Verification items for the finished model (mm, model axes). Coordinates: 2 decimals unless noted, no trailing zeros. Order: outer loops, then holes, each group sorted by start corner. A loop starts at its lowest first (then second) coordinate and runs counter-clockwise, first axis right, second up. Notation, with made-up numbers: M -24.5,-14.5 L 14.5,-14.5 A15 cw 14.5,10.5 Z; hole C -18.5,-26.5 d6. An arc over 180 degrees is marked long. Return JSON: item names as keys, results as strings. Group by question number.
1. Material ranges on line 1 along Y through (x, z) = (2, 17); line 2 along Y through (x, z) = (-54.5, 13.25); line 3 along Y through (x, z) = (-155.5, 5.5), recorded low to high.
2. Section check D-D, the plane x = 74. Record the cut outline in (y, z), plus the area to 3 significant figures.
3. Section check C-C, the plane x = 7. Record the cut outline in (y, z).
4. Section check A-A, the plane z = 10.5. Record the cut outline in (x, y).
5. Gauge pin test, flat end, axial feed: pin 1 (4 mm diameter, centred on x = -7, z = 16.5, fed in from -Y). Record the tip position at first contact, or that the pin passes through.
6. Section check B-B, the plane y = 96.5. Record the cut outline in (x, z), plus the area to 3 significant figures.
```python
from build123d import *

# Parameters (mm, degrees)
F0_W     = 400
F0_H     = 350
F1_DEPTH = 19
F2_W     = 400
F2_H     = 350
F3_DEPTH = 19.001
F5_DEPTH = 19.001


with BuildPart() as f1:
    # F0 (on Top) → F1 (new body)
    with BuildSketch(Plane.XY):
        with Locations((0, -4.671676)):
            Rectangle(F0_W, F0_H)
    extrude(amount=F1_DEPTH)

    # F2 (on face) → F3 (cut, through all)
    with BuildSketch(Plane.XY.offset(19)):
        with Locations((0, -4.671676)):
            Rectangle(F2_W, F2_H)
        with BuildLine():
            ThreePointArc((192.000002, -145.333663), (0.340362, -123.303121), (-191.445097, -144.210055))
            Line((-191.445097, -144.210055), (-191.445097, 137.21716))
            ThreePointArc((-191.445097, 137.21716), (0.366935, 114.931669), (192.000002, 138.707012))
            Line((192.000002, 138.707012), (192.000002, -145.333663))
        make_face(mode=Mode.SUBTRACT)
    extrude(amount=-F3_DEPTH, mode=Mode.SUBTRACT)

    # F4 (on face) → F5 (cut, through all)
    with BuildSketch(Plane.XY.offset(19)):
        with BuildLine():
            ThreePointArc((56.528851, 112.057194), (-3.020095, 108.082536), (-62.591754, 111.70088))
            Line((-62.591754, 111.70088), (-62.591754, 88.262614))
            ThreePointArc((-62.591754, 88.262614), (-3.075748, 80.144421), (56.528851, 87.584293))
            Line((56.528851, 87.584293), (56.528851, 112.057194))
        make_face()
    extrude(amount=-F5_DEPTH, mode=Mode.SUBTRACT)


solid = f1.part
```
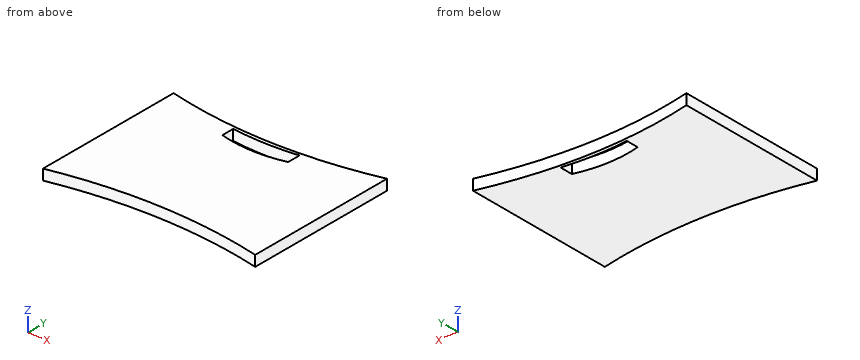
Answers follow:
{
 "1": {"line 1": "-123.31 to 80.17, 108.12 to 114.94", "line 2": "-124.88 to 86.22, 110.76 to 116.58", "line 3": "-136.96 to 129.46"},
 "2": {"outline": "M -126.66,0 L 118.57,0 L 118.57,19 L -126.66,19 Z", "area": "4,660 mm^2"},
 "3": {"outline": "M -123.35,0 L 80.31,0 L 80.31,19 L -123.35,19 Z; M 108.22,0 L 114.98,0 L 114.98,19 L 108.22,19 Z"},
 "4": {"outline": "M -191.45,-144.21 A866.81 cw 192,-145.33 L 192,138.71 A809.54 cw -191.45,137.22 Z; hole M -62.59,88.26 A231.91 ccw 56.53,87.58 L 56.53,112.06 A469.1 cw -62.59,111.7 Z"},
 "5": {"pin 1": "y = -123.33"},
 "6": {"outline": "M -191.45,0 L -62.59,0 L -62.59,19 L -191.45,19 Z; M 56.53,0 L 192,0 L 192,19 L 56.53,19 Z", "area": "5,020 mm^2"}
}
